Geometry: final body of the model. Coordinates: model frame, mm. Give positions to 0.01 mm unless a question says otherwise; leave off trailing zeros. Write each loop counter-clockwise with the first axis right and the second up, starting at its lowest first coordinate (ties: lowest second). Pieces come first, ordered by that corner, then holes.
from build123d import *

# Parameters (mm, degrees)
ESQUISSE1_W = 7
ESQUISSE1_H = 7
CONG_1_R    = 0.5


with BuildPart() as part:
    # Esquisse1 → Révolution1 (revolve)
    with BuildSketch(Plane.XY):
        with Locations((7.5, 3.5)):
            Rectangle(ESQUISSE1_W, ESQUISSE1_H)
    revolve(axis=Axis((0, 0, 0), (0, 1, 0)))

    # Congé1
    cong_1_edges = [part.edges().sort_by_distance(p)[0] for p in [
        (-4, 0, 0),
        (-11, 0, 0),
        (-11, 7, 0),
        (-4, 7, 0),
    ]]
    fillet(cong_1_edges, radius=CONG_1_R)


solid = part.part
Q1. Pin query (flat end, axial travel): P1, Ø3, axis at x = -2, y = 2.5, coming from the +Z side; P2, Ø1.5, axis at x = 2, z = -3, coming from the +Y side. Return the tip coordinate at first contact, or that it passes through.
Filled sheet:
P1: stops at z = 10.99
P2: stops at y = 6.98
Q2. Pull-direction query (X, two-part tool) for faces 1 (the cylindrical face through (-0.867, 3.542, 3.905)), 2 (the cylindrical face through (-2.38, 3.54, 10.74)), 3 (the flat face through (-5, 0, 0)); classes: released by +X, released by -X, zero draft, split by the parting line, or undercut.
Filled sheet:
face 1: undercut
face 2: split by the parting line
face 3: zero draft
Q3. Ray query, line 1 along X through (y, z) = (4.6, 0); line 2 along X through (y, z) = (3.25, -1.25). Return the intervals inside material, ascending.
Filled sheet:
line 1: x = -11 to -4, 4 to 11
line 2: x = -10.93 to -3.8, 3.8 to 10.93
Q4. Section A-A on x = 0. Output: boundary loops of the cut face in (y, z), plus the area to 3 significant figures.
Filled sheet:
outline: (0, -10.5) arc R0.5 ccw to (0.5, -11) - (6.5, -11) arc R0.5 ccw to (7, -10.5) - (7, -4.5) arc R0.5 ccw to (6.5, -4) - (0.5, -4) arc R0.5 ccw to (0, -4.5) - close; (0, 4.5) arc R0.5 ccw to (0.5, 4) - (6.5, 4) arc R0.5 ccw to (7, 4.5) - (7, 10.5) arc R0.5 ccw to (6.5, 11) - (0.5, 11) arc R0.5 ccw to (0, 10.5) - close
area: 97.6 mm2
Q5. Section B-B on z = 0. Output: boundary loops of the cut face in (x, y).
Filled sheet:
outline: (-11, 0.5) arc R0.5 ccw to (-10.5, 0) - (-4.5, 0) arc R0.5 ccw to (-4, 0.5) - (-4, 6.5) arc R0.5 ccw to (-4.5, 7) - (-10.5, 7) arc R0.5 ccw to (-11, 6.5) - close; (4, 0.5) arc R0.5 ccw to (4.5, 0) - (10.5, 0) arc R0.5 ccw to (11, 0.5) - (11, 6.5) arc R0.5 ccw to (10.5, 7) - (4.5, 7) arc R0.5 ccw to (4, 6.5) - close
Q6. Section C-C on y = 4. Output: boundary loops of the cut face in (x, z).
Filled sheet:
outline: circle Ø22 at (0, 0); hole circle Ø8 at (0, 0)
